Read the model definition and answer for the solid it produces. Units are mm, in the model's axes. A direction names the side the tool comes from. Round coordinates to 2 decimals unless told otherwise and drop trailing zeros. Order: outer loops, then holes, each group sorted by start corner. A loop starts at its lowest first (then second) coordinate and runs counter-clockwise, first axis right, second up. Notation, with made-up numbers: (81, 35.5) - (99, 35.5) arc R18 cw to (99, 57.5) - close; hole circle Ø3 at (-29.75, -13). An arc over 180 degrees is marked (long way). Answer as a JSON object with one key per item and string values. Group by question number.
Q1. A cutting plane is placed at C-C on y = -44. Determine the outline of the cut face in (x, z), and give its area (3 significant figures).
Q2. A cutting plane is placed at B-B on z = 0. Determine the outline of the cut face in (x, y), and give its area (3 significant figures).
Q3. A tool of negligible diameter and unlimited length cuts with its end or side. For faces 4 (the cylindrical face through (-14.85, -5.04, 66.87)), 5 (the flat face through (37, -10, -58)), 6 (the cylindrical face through (0, -1, -50)), from which of +Z, -Z, +X, -X, +Y, -Y can it reach the whole face along a straight path? Write none if from no direction.
Q4. A cutting plane is placed at A-A on x = 0. Count the separate pieces of the cut face and the enclosed holes in it, and give its area (3 significant figures).
Q5. Given pin 1 Ø12 at (x, z) = (-41, 3.5) entering from -Y; pin 2 Ø5 at (y, z) = (-37, 6.5) entering from +X; pin 3 Ø1 at (y, z) = (-9, -44) entering from -X, each flat-ended and moving along its own axis, determine where each tip first touches the part or whether it passes through.
Q6. The mould has two halves that part along Y. Classify faces 1 (the cylindrical face through (-4.88, -0.99, -1.08)), 2 (the flat face through (-36, -8, -56)), 3 (the flat face through (14, 0, -1)): pulls with the +Y half, pulls with the -Y half, needs draft (parallel to the pull), parting line crosses it, or undercut.
Q7. Consider line 1 (Z direction, x = 0, y = -17.5); line 2 (Y direction, x = 3, z = -64); line 3 (X direction, y = -10.5, z = 26.5). Determine where each line is inside the solid, lowest interval first.
```python
from build123d import *

# Parameters (mm, degrees)
SVUOTA5_START            = -60
SVUOTA5_OUTLINE_R        = 66
SVUOTA5_DEPTH            = 58
SVUOTA5_START_2          = -8
SVUOTA5_2_OUTLINE_R      = 68.499999813
SVUOTA5_2_OUTLINE_R_2    = 66
SVUOTA5_2_DEPTH          = 6
SMUSSO1_SIZE             = 2
SCHIZZO3_R               = 5
TAGLIO_ESTRUSIONE1_DEPTH = 10
SCHIZZO4_R               = 5
TAGLIO_ESTRUSIONE2_DEPTH = 10


# Read off the part's stored shape, not the designer's step: Svuota5
with BuildPart() as part:
    # Schizzo1 → Rivoluzione3 (revolve)
    with BuildSketch(Plane.XY):
        with BuildLine():
            Line((0, 0), (0, -10))
            Line((0, -10), (0, -60))
            Line((0, -60), (66, -60))
            ThreePointArc((66, -60), (67.414213562, -59.414213562), (68, -58))
            Line((68, -58), (68, -10))
            Line((68, -10), (70.499999813, -10))
            Line((70.499999813, -10), (70.499999813, 0))
            Line((70.499999813, 0), (0, 0))
        make_face()
    revolve(axis=Axis((0, -60, 0), (0, 1, 0)))

    # Svuota5 outline → Svuota5 (cut)
    with BuildSketch(Plane(origin=(0, 0, 0), x_dir=(1, 0, 0), z_dir=(0, 1, 0)).offset(SVUOTA5_START)):
        Circle(SVUOTA5_OUTLINE_R)
    extrude(amount=SVUOTA5_DEPTH, mode=Mode.SUBTRACT)

    # Svuota5 2 outline → Svuota5 2 (cut)
    with BuildSketch(Plane(origin=(0, 0, 0), x_dir=(1, 0, 0), z_dir=(0, 1, 0)).offset(SVUOTA5_START_2)):
        Circle(SVUOTA5_2_OUTLINE_R)
        Circle(SVUOTA5_2_OUTLINE_R_2, mode=Mode.SUBTRACT)
    extrude(amount=SVUOTA5_2_DEPTH, mode=Mode.SUBTRACT)

    # Smusso1
    smusso1_edges = [part.edges().sort_by_distance(p)[0] for p in [
        (-70.499999813, 0, 0),
    ]]
    chamfer(smusso1_edges, length=SMUSSO1_SIZE)

    # Schizzo3 → Taglio-Estrusione1 (cut)
    with BuildSketch(Plane(origin=(0, 0, 0), x_dir=(1, 0, 0), z_dir=(0, 1, 0))):
        with Locations(Location((0, 0, 0), (0, 0, 270))):
            Circle(SCHIZZO3_R)
    extrude(amount=-TAGLIO_ESTRUSIONE1_DEPTH, mode=Mode.SUBTRACT)

    # Schizzo4 → Taglio-Estrusione2 (cut)
    with BuildSketch(Plane(origin=(0, 0, 0), x_dir=(1, 0, 0), z_dir=(0, 1, 0))):
        with Locations(Location((0, 45, 0), (0, 0, 270))):
            Circle(SCHIZZO4_R)
        with Locations(Location((0, -45, 0), (0, 0, 270))):
            Circle(SCHIZZO4_R)
    extrude(amount=-TAGLIO_ESTRUSIONE2_DEPTH, mode=Mode.SUBTRACT)


solid = part.part
```
Result set:
{
 "1": {"outline": "circle Ø136 at (0, 0); hole circle Ø132 at (0, 0)", "area": "842 mm²"},
 "2": {"outline": "(-70.5, -10) - (-68, -10) - (-68, -58) arc R2 ccw to (-66, -60) - (-66, -8) - (-68.5, -8) - (-68.5, -2) - (-5, -2) - (-5, 0) - (-68.5, 0) - (-70.5, -2) - close; (5, -2) - (68.5, -2) - (68.5, -8) - (66, -8) - (66, -60) arc R2 ccw to (68, -58) - (68, -10) - (70.5, -10) - (70.5, -2) - (68.5, 0) - (5, 0) - close", "area": "498 mm²"},
 "3": {"face 4": "none", "face 5": "-Y", "face 6": "+Y, -Y"},
 "4": {"separate pieces": "4", "enclosed holes": "0", "area": "458 mm²"},
 "5": {"pin 1": "stops at y = -2", "pin 2": "stops at x = 67.88", "pin 3": "stops at x = -55.48"},
 "6": {"face 1": "needs draft", "face 2": "undercut", "face 3": "pulls with the +Y half"},
 "7": {"line 1": "z = -68 to -66, 66 to 68", "line 2": "y = -2 to 0", "line 3": "x = -62.62 to -60.45, 60.45 to 62.62"}
}
